Can you work these out from the drawing? Everything is in mm from the part's minimum corner. Give positions to 0.01 mm unless a question says otherwise; leave off trailing zeros. Order: outer loops, then holes, each group sorted by start corner. A loop starts at its lowest first (then second) coordinate and runs counter-clockwise, first axis right, second up. Notation, with made-up numbers: (51.5, -5) -> (70.5, -5) arc R17 ccw to (70.5, 7) -> close; hole circle Ø8 at (77.5, 6). An arc over 180 degrees is marked (long way). One line per item, written item: value.
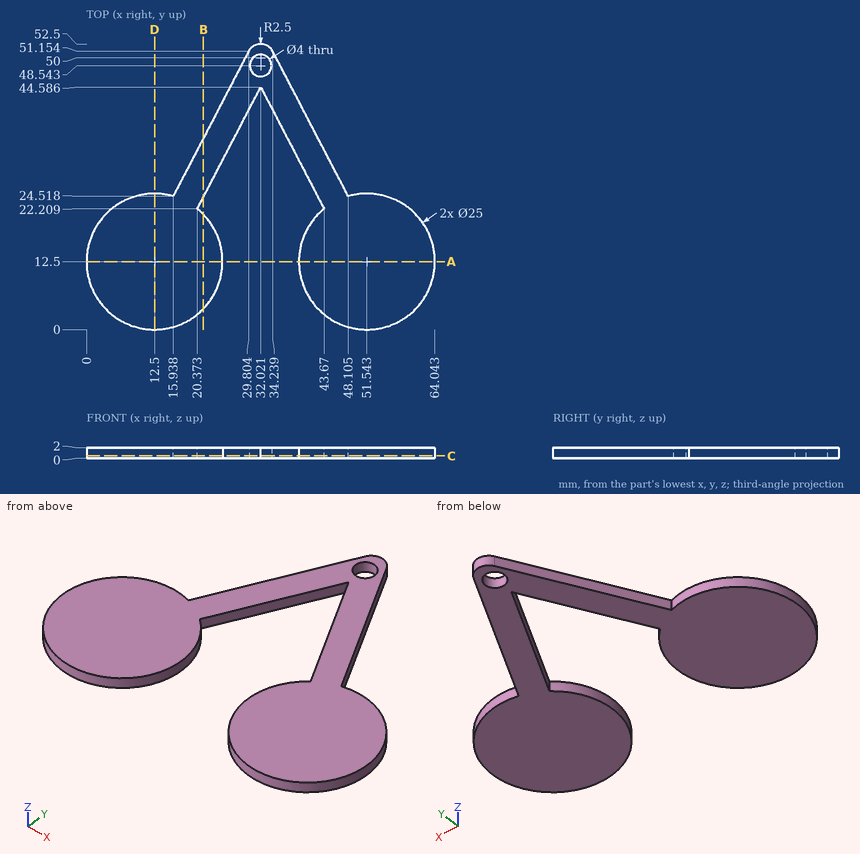
1) If I drill on line 1 along X through (y, z) = (17, 1.1) (1 decimal); line 2 along X through (y, z) = (27, 1.3) (1 decimal); line 3 along Y through (x, z) = (31, 0.7) (1 decimal), over which ranges is the centre line in solid material (lowest first)?
Answer below:
line 1: x = 0.8 to 24.2, 39.9 to 63.2
line 2: x = 17.2 to 22.9, 41.2 to 46.8
line 3: y = 42.6 to 46.8, 50.3 to 52.3
2) Suppose I cut it at A-A, the plane y = 12.5. Write out the boundary of the cut face in (x, z).
Answer below:
outline: (0, 0) -> (25, 0) -> (25, 2) -> (0, 2) -> close; (39.04, 0) -> (64.04, 0) -> (64.04, 2) -> (39.04, 2) -> close
3) Suppose I cut it at D-D, the plane x = 12.5. Write out the boundary of the cut face in (y, z).
Answer below:
outline: (0, 0) -> (25, 0) -> (25, 2) -> (0, 2) -> close
4) Suppose I cut it at C-C, the plane z = 0.5. Write out the boundary of the cut face in (x, y) (1 decimal), then the cut area to 3 significant figures.
Answer below:
outline: (15.9, 24.5) arc R12.5 ccw (long way) to (20.4, 22.2) -> (32, 44.6) -> (43.7, 22.2) arc R12.5 ccw (long way) to (48.1, 24.5) -> (34.2, 51.2) arc R2.5 ccw to (29.8, 51.2) -> close; hole circle Ø4 at (32, 48.5)
area: 1,260 mm2
5) Suppose I cut it at B-B, the plane x = 21.5. Write out the boundary of the cut face in (y, z) (1 decimal).
Answer below:
outline: (3.8, 0) -> (21.2, 0) -> (21.2, 2) -> (3.8, 2) -> close; (24.4, 0) -> (35.2, 0) -> (35.2, 2) -> (24.4, 2) -> close
6) For P1, Ø2.5, axis at x = 32.02, y = 48.54, coming from the -Z side, with a flat end and sliding along its axis, tell me the tip position at first contact or that it passes through.
Answer below:
P1: passes through
